Work out the finished part from the listing and answer in its coordinate system (mm). Face numbers are marked on the shaded views. A direction names the side the tool comes from. Give positions to 0.01 mm unless a question says otherwise; leave off trailing zeros. Write each loop counter-clockwise with the first axis right and the second up, starting at its lowest first coordinate (ties: lowest second). Pieces come first, ordered by that corner, then holes.
1) Find section B-B (x = 384). Determine the outline of the cut face in (y, z), plus the area to 3 significant figures.
2) Straight lines are drawn through the part: probe 1 along Y at (x, z) = (96, 10.5); probe 2 along Y at (x, z) = (303, 7.5); probe 3 along X at (y, z) = (126.5, 38.5). For each, find the intervals that lie inside material, in ascending order.
3) A tool of negligible diameter and unlimited length cuts with its end or side. For the marked faces 1 and 2, from which of +Z, -Z, +X, -X, +Y, -Y can it reach the whole face along a straight path? Write none if from no direction.
4) Determine the mould class of the marked faces 3, 4 and 5 for opening direction Y: pulls with the +Y half, pulls with the -Y half, needs draft (parallel to the pull), parting line crosses it, or undercut.
5) Find section A-A (z = 30). Determine the outline of the cut face in (x, y).
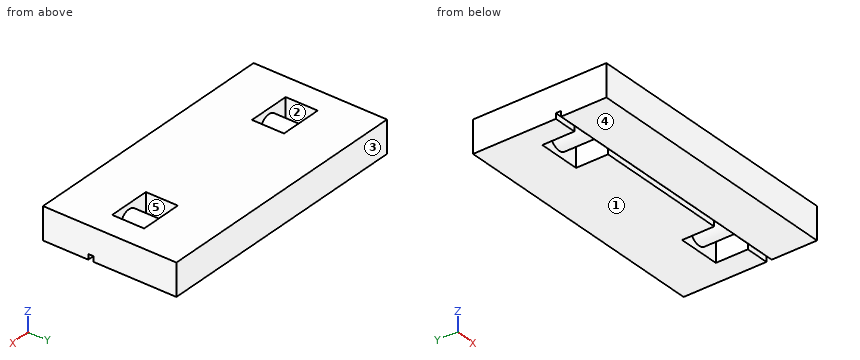
```python
from build123d import *

# Parameters (mm, degrees)
SKETCH_1_W          = 500
SKETCH_1_H          = 250
EXTRUDE_1_DEPTH     = 60
SKETCH_5_W          = 10
SKETCH_5_H          = 10
CUT_EXTRUDE_3_DEPTH = 500
CUT_EXTRUDE_START   = -94.842468
SKETCH_2_R          = 20
CUT_EXTRUDE_4_DEPTH = 60


with BuildPart() as part:
    # 草图1 → 凸台-拉伸1 (new body)
    with BuildSketch(Plane.XY):
        with Locations((250, 125)):
            Rectangle(SKETCH_1_W, SKETCH_1_H)
    extrude(amount=EXTRUDE_1_DEPTH)

    # 草图5 → 切除-拉伸3 (cut)
    with BuildSketch(Plane(origin=(0, 0, 0), x_dir=(0, 0, -1), z_dir=(1, 0, 0))):
        with Locations((-5, 89.842468298)):
            Rectangle(SKETCH_5_W, SKETCH_5_H)
    extrude(amount=CUT_EXTRUDE_3_DEPTH, mode=Mode.SUBTRACT)

    # 草图2 → 切除-拉伸4 (cut)
    # profile 1 of 2: a face of its own
    with BuildSketch(Plane.XZ.offset(CUT_EXTRUDE_START)):
        Polygon((100, 60), (124, 60), (124, 0), (44, 0), (44, 60), align=None)
        with Locations(Location((84, 30, 0), (0, 0, 270))):
            Circle(SKETCH_2_R, mode=Mode.SUBTRACT)
    # profile 2 of 2: a face of its own
    with BuildSketch(Plane.XZ.offset(CUT_EXTRUDE_START)):
        Polygon((456, 60), (400, 60), (376, 60), (376, 0), (456, 0), align=None)
        with Locations(Location((416, 30, 0), (0, 0, 270))):
            Circle(SKETCH_2_R, mode=Mode.SUBTRACT)
    extrude(amount=-CUT_EXTRUDE_4_DEPTH, mode=Mode.SUBTRACT)


solid = part.part
```
Results:
1. outline: (0, 0) - (84.84, 0) - (84.84, 10) - (94.84, 10) - (94.84, 60) - (0, 60) - close; (154.84, 0) - (250, 0) - (250, 60) - (154.84, 60) - close
1. area: 11,300 mm2
2. probe 1: y = 0 to 94.84, 154.84 to 250
2. probe 2: y = 0 to 84.84, 94.84 to 250
2. probe 3: x = 0 to 44, 65.9 to 102.1, 124 to 376, 397.9 to 434.1, 456 to 500
3. face 1: -Z, +X, -X, +Y, -Y
3. face 2: +Z, -Z
4. face 3: pulls with the +Y half
4. face 4: needs draft
4. face 5: undercut
5. outline: (0, 0) - (500, 0) - (500, 250) - (0, 250) - close; hole (44, 94.84) - (64, 94.84) - (64, 154.84) - (44, 154.84) - close; hole (104, 94.84) - (124, 94.84) - (124, 154.84) - (104, 154.84) - close; hole (376, 94.84) - (396, 94.84) - (396, 154.84) - (376, 154.84) - close; hole (436, 94.84) - (456, 94.84) - (456, 154.84) - (436, 154.84) - close
